from build123d import *

# Parameters (mm, degrees)
MAIN_DEPTH          = 5
SKETCH2_R           = 1.25
FIXHOLE1_DEPTH      = 84
SKETCH3_R           = 1.25
FIXHOLE2_DEPTH      = 84
SKETCH6_R           = 1.25
CUT_EXTRUDE2_DEPTH  = 64.639610307
LPATTERN1_COUNT     = 5
LPATTERN1_PITCH     = 20
SKETCH7_R           = 5
BOSS_EXTRUDE1_DEPTH = 3
SKETCH8_R           = 1.25
CUT_EXTRUDE3_DEPTH  = 67.639610307


with BuildPart() as part:
    # Sketch1 → Main (new body, symmetric)
    with BuildSketch(Plane.XY):
        Polygon((-41.5, -41.5), (41.5, 41.5), (41.5, 39.5), (51.5, 39.5), (51.5, 34.5), (41.5, 34.5), (-34.5, -41.5), (-34.5, -51.5), (-39.5, -51.5), (-39.5, -41.5), align=None)
    extrude(amount=MAIN_DEPTH, both=True)

    # Sketch2 → FixHole1 (cut, through all)
    with BuildSketch(Plane(origin=(41.5, 0, 0), x_dir=(0, 0, -1), z_dir=(1, 0, 0))):
        with Locations((0, -46.5)):
            Circle(SKETCH2_R)
    extrude(amount=-FIXHOLE1_DEPTH, mode=Mode.SUBTRACT)

    # Sketch3 → FixHole2 (cut, through all)
    with BuildSketch(Plane(origin=(0, -41.5, 0), x_dir=(-1, 0, 0), z_dir=(0, -1, 0))):
        with Locations((-46.5, 0)):
            Circle(SKETCH3_R)
    extrude(amount=-FIXHOLE2_DEPTH, mode=Mode.SUBTRACT)

    # Sketch6 → Cut-Extrude2 (cut, through all)
    with BuildSketch(Plane(origin=(3.5, -3.5, 0), x_dir=(0, 0, 1), z_dir=(-0.707106781, 0.707106781, 0))):
        with Locations((0, 40)):
            Circle(SKETCH6_R)
    cut_extrude2 = extrude(amount=CUT_EXTRUDE2_DEPTH, mode=Mode.SUBTRACT)

    # LPattern1: Cut-Extrude2 ×5
    with Locations(*[Vector(-0.707106781, -0.707106781, 0) * (i * LPATTERN1_PITCH) for i in range(1, LPATTERN1_COUNT)]):
        add(cut_extrude2, mode=Mode.SUBTRACT)

    # Sketch7 → Boss-Extrude1 (add)
    with BuildSketch(Plane(origin=(3.5, -3.5, 0), x_dir=(0, 0, 1), z_dir=(-0.707106781, 0.707106781, 0))):
        with Locations((0, -32.4)):
            Circle(SKETCH7_R)
        with Locations((0, 32.4)):
            Circle(SKETCH7_R)
    extrude(amount=-BOSS_EXTRUDE1_DEPTH)

    # Sketch8 → Cut-Extrude3 (cut, through all)
    with BuildSketch(Plane(origin=(5.621320344, -5.621320344, 0), x_dir=(0, 0, -1), z_dir=(0.707106781, -0.707106781, 0))):
        with Locations((0, 32.4)):
            Circle(SKETCH8_R)
        with Locations((0, -32.4)):
            Circle(SKETCH8_R)
    extrude(amount=-CUT_EXTRUDE3_DEPTH, mode=Mode.SUBTRACT)


solid = part.part
Can you work these out from the model? Positions are in its coordinate system, mm. A direction names the side the tool comes from. Round coordinates to 2 decimals unless told otherwise and drop trailing zeros. Loops run counter-clockwise (first coordinate to the right, second up) from the corner with the lowest first, then second, coordinate; pieces in that order, holes last. Notation, with made-up numbers: (88, 33) - (140, 33) arc R9 cw to (140, 38) - close; hole circle Ø9 at (-30, 58.25). An arc over 180 degrees is marked (long way). Write item = value, one per line. Start each with the question number.
(1) If we section it at A-A (x = 46.5): Please give me the cut outline in (y, z).
(2) If we mould it in two halves opening along X, with no side actions, what happens to faces 6 (the face through (24.897, 19.197, 0.271)), 7 (the face through (2, -1, 5)), 8 (the face through (51.5, 37, 0))? For each: released by +X, released by -X, zero draft, split by the parting line, or undercut.
(3) If we section it at D-D (y = -12): Please give me the cut outline in (x, z), and give its area (3 significant figures).
(4) If I drill on probe 1 along Z at (x, y) = (46.5, 37.9); probe 2 along X at (y, z) = (-44.5, 2.5); probe 3 along Y at (x, z) = (-37.5, 0), over which ranges is the centre line in solid material (lowest first)? Write a range as [from, to].
(5) For faces 1 (the face through (-19.184, -24.884, 0.163)), 2 (the face through (48, 39.5, 1)), 3 (the face through (-36.97, -45.26, 0.16)), 4 (the face through (-40, -41.5, 0)), 5 (the face through (-34.5, -48, 1)), which set-ups out of +Z, -Z, +X, -X, +Y, -Y let a thin tool reach every point of the face, with its end or its side?
(6) For P1, Ø2, axis at x = 5, z = 3.5, coming from the +Y side; P2, Ø4, axis at x = 46.5, z = 0, coming from the +Y side; P3, Ø5, axis at x = -1, z = 0.5, coming from the -Y side, each with a flat end and sliding along its axis, tell me the tip position at first contact or that it passes through.
(7) If we section it at C-C (z = 3.5): Please give me the cut outline in (x, y), and give its area (3 significant figures).
(8) If we section it at B-B (y = -46.5): Please give me the cut outline in (x, z).
Ans:
q1.outline = (34.5, -5) - (39.5, -5) - (39.5, -1.25) - (34.5, -1.25) - close; (34.5, 1.25) - (39.5, 1.25) - (39.5, 5) - (34.5, 5) - close
q2.face_6 = undercut
q2.face_7 = zero draft
q2.face_8 = released by +X
q3.outline = (-12, -5) - (-5, -5) - (-5, 5) - (-12, 5) - close
q3.area = 70.0 mm²
q4.probe_1 = [-5, -1.25], [1.25, 5]
q4.probe_2 = [-39.5, -34.5]
q4.probe_3 = [-51.5, -47.75], [-45.25, -37.5]
q5.face_1 = none
q5.face_2 = +Z, -Z, +X, +Y
q5.face_3 = +X, -X
q5.face_4 = +Z, -Z, -X, -Y
q5.face_5 = +Z, -Z, +X, -Y
q6.P1 = 6
q6.P2 = 39.5
q6.P3 = -10.5
q7.outline = (-41.5, -41.5) - (-39.5, -41.5) - (-39.5, -51.5) - (-34.5, -51.5) - (-34.5, -41.5) - (-21.94, -28.94) - (-19.81, -31.06) - (-14.76, -26.01) - (-16.89, -23.89) - (23.89, 16.89) - (26.01, 14.76) - (31.06, 19.81) - (28.94, 21.94) - (41.5, 34.5) - (51.5, 34.5) - (51.5, 39.5) - (41.5, 39.5) - (41.5, 41.5) - close
q7.area = 699 mm²
q8.outline = (-39.5, -5) - (-34.5, -5) - (-34.5, -1.25) - (-39.5, -1.25) - close; (-39.5, 1.25) - (-34.5, 1.25) - (-34.5, 5) - (-39.5, 5) - close
